The model under review builds one solid part; all positions refer to its coordinate system, in mm. A direction names the side the tool comes from. Coordinates: 2 decimals unless noted, no trailing zeros. Write each loop counter-clockwise with the first axis right and the second up, starting at its lowest first coordinate (ties: lowest second). Pieces come first, ordered by that corner, then holes.
1) For P1, Ø4, axis at x = 0, z = 1, coming from the +Y side; P2, Ø8, axis at y = -10, z = 3.5, coming from the +X side; P3, Ø1.2, axis at x = 0.5, z = 0.5, coming from the +Y side; P4, Ø1.6, axis at x = 0, z = 0, coming from the -Y side, all flat-tipped, find the tip position at first contact; note any pin that passes through.
2) For line 1 (Z direction, x = 0, y = 4.75); line 2 (Y direction, x = -4.75, z = -2.5); line 3 (X direction, y = 2.75, z = -1), list the stretches that pass through material, from the lowest coordinate up.
3) Add section B-B, the plane y = -2.25. State the section outline as (x, z) points (3 decimals), then the cut area to 3 significant figures.
4) Add section C-C, the plane z = 2.75. State the section outline as (x, y) points, then the cut area to 3 significant figures.
5) Add section D-D, the plane x = -3.25. State the section outline as (y, z) points, then the cut area to 3 significant figures.
6) Add section A-A, the plane z = 0. State the section outline as (x, y) points.
7) Machinability: for faces 1 (the flat face through (2, -5, -5)), 2 (the cylindrical face through (0, -5, -2)), 3 (the flat face through (7, -2, 0)), which of the approach directions +Z, -Z, +X, -X, +Y, -Y give a long, thin tool a straight path to every point of the face, cutting with its end or side? Answer none if there is none.
8) Mouldability with a two-part tool opening along X and no side actions: class faces 4 (the cylindrical face through (-1.08, -8.55, -4.88)), 5 (the flat face through (-3.557, -2.465, 5.416)), 6 (the flat face through (2, 7, 2)), 7 (the flat face through (1, -10, -1)) as released by +X, released by -X, zero draft, split by the parting line, or undercut.
Autodesk Inventor part; units mm, degrees
ref_plane "YZ Plane" through (0, 0, 0) normal (1, 0, 0) x (0, 1, 0)
ref_plane "XZ Plane" through (0, 0, 0) normal (0, 1, 0) x (-1, 0, 0)
ref_plane "XY Plane" through (0, 0, 0) normal (0, 0, 1) x (1, 0, 0)
sketch "Boceto1" plane through (0, 0, 0) normal (0, 0, 1) x (1, 0, 0)
  line L0 (0, 9.3809) -> (0, -9.3809)
  line L1 (-19.2892, 0) -> (19.2892, 0) construction
  line L2 (0, 7) -> (4, 7)
  line L3 (4, 0) -> (4, 7)
  line L4 (4, 0) -> (7, 0)
  line L5 (7, 0) -> (7, -5)
  line L6 (7, -5) -> (0, -5)
  line L7 (5, -5) -> (5, -12)
  line L8 (5, -12) -> (0, -12)
  line L9 (2.5, 7) -> (2.5, 0)
  line L10 (2, -5) -> (2, -10)
  line L11 (2.5, 0) -> (2.5, -0.5101)
  line L12 (2.5, -0.5101) -> (2, -0.5101)
  line L13 (2, -5) -> (2, -0.5101)
  line L14 (2, -10) -> (1, -10)
  line L15 (1, -10) -> (1, -12)
  point P0 (0, 0)
  point P1 (0, 0)
  dimension "d0" = 14
  dimension "d1" = 10
  dimension "d2" = 8
  dimension "d3" = 5
  dimension "d4" = 4
  dimension "d5" = 2
  dimension "d6" = 2
  dimension "d7" = 7
  dimension "d8" = 5
  dimension "d9" = 7
revolve "Revolución1" add sketch "Boceto1" angle 360 about axis through (0, 9.3809, 0) along (0, -1, 0) contours L2 L3 L4 L5 L6 L13 L12 L11 L9 | L6 L7 L8 L15 L14 L10
sketch "Boceto2" plane through (0, 0, 0) normal (0, 1, 0) x (1, 0, 0)
  circle A0 centre (0, 0) radius 2.5
  circle A1 centre (0, 0) radius 4
  circle A2 centre (0, 0) radius 4
  circle A3 centre (0, 0) radius 7
  line L0 (7, 3.875) -> (7, -3.875)
  line L1 (-7, 3.875) -> (-7, -3.875)
  circle A4 centre (0, 0) radius 7
  line L2 (-7, 3.875) -> (0.0154, 7)
  line L3 (0.0154, 7) -> (7, 3.875)
  line L4 (-7, -3.875) -> (-0.0154, -7)
  line L5 (-0.0154, -7) -> (7, -3.875)
  arc A5 (0.0154, 7) -> (-5.214, 4.6706) centre (0, 0) ccw
  circle A6 centre (0, 0) radius 7
  arc A7 (5.2088, 4.6764) -> (0.0154, 7) centre (0, 0) ccw
  arc A8 (-0.0154, -7) -> (5.214, -4.6706) centre (0, 0) ccw
  arc A9 (-5.2088, -4.6764) -> (-0.0154, -7) centre (0, 0) ccw
  point P0 (0, 0)
  point P1 (7, 0)
  point P2 (-7, 0)
  point P3 (-0.0154, -7)
  point P4 (-0.0154, -7)
  point P5 (-5.2088, -4.6764)
  point P6 (5.214, -4.6706)
  point P7 (5.2088, 4.6764)
  point P8 (-5.214, 4.6706)
  dimension "d15" = 14
  dimension "d27" = 7.75
  dimension "d28" = 14
  dimension "d29" = 14
  dimension "d30" = 7.75
  dimension "d51" = 7
  dimension "d52" = 1.786
  dimension "d53" = 1.7913
  dimension "d54" = 7.0154
  dimension "d55" = 7.0154
  dimension "d56" = 12.7918
  dimension "d57" = 12.2088
  dimension "d58" = 12.7918
  dimension "d59" = 12.214
  dimension "d60" = 4.2619
  dimension "d61" = 7
  dimension "d62" = 7
  dimension "d63" = 7
extrude "Extrusión1" cut sketch "Boceto2" against normal through all contours L3 A3 | A3 L5 | L2 A3 | A3 L4
extrude "Extrusión2" add sketch "Boceto2" against normal blind 5 contours L0 L5 A3 | A3 L3 L0 | A3 L1 L2 | L4 L1 A3
thread "Rosca2"
thread "Rosca3"
equation "\"d30\" = d27"
properties part number "1-HUDSON-8-29-TDR HAND PUMP BODY TOP OUTLET"
Geometry results:
1. P1: stops at y = 7
1. P2: stops at x = 5
1. P3: stops at y = -10
1. P4: passes through
2. line 1: z = -4 to -2.5, 2.5 to 4
2. line 2: y = -5 to 0
2. line 3: x = -3.87 to -2.29, 2.29 to 3.87
3. outline: (-7, -3.875) - (0.015, -7) - (7, -3.875) - (7, 3.875) - (-0.015, 7) - (-7, 3.875) - close; hole circle Ø4 at (0, 0)
3. area: 140 mm2
4. outline: (-7, -5) - (-4.18, -5) - (-4.18, -12) - (4.18, -12) - (4.18, -5) - (7, -5) - (7, 0) - (2.9, 0) - (2.9, 7) - (-2.9, 7) - (-2.9, 0) - (-7, 0) - close
4. area: 169 mm2
5. outline: (-12, -3.8) - (-5, -3.8) - (-5, -5.55) - (0, -5.55) - (0, -2.33) - (7, -2.33) - (7, 2.33) - (0, 2.33) - (0, 5.55) - (-5, 5.55) - (-5, 3.8) - (-12, 3.8) - close
5. area: 141 mm2
6. outline: (-7, -5) - (-5, -5) - (-5, -12) - (-1, -12) - (-1, -10) - (-2, -10) - (-2, -0.51) - (-2.5, -0.51) - (-2.5, 7) - (-4, 7) - (-4, 0) - (-7, 0) - close; (1, -12) - (5, -12) - (5, -5) - (7, -5) - (7, 0) - (4, 0) - (4, 7) - (2.5, 7) - (2.5, -0.51) - (2, -0.51) - (2, -10) - (1, -10) - close
7. face 1: -Y
7. face 2: +Y
7. face 3: +Z, -Z, +X, +Y, -Y
8. face 4: split by the parting line
8. face 5: released by -X
8. face 6: zero draft
8. face 7: undercut
